Can you work these out from the model? Positions are in its coordinate system, mm. A direction names the side the tool comes from. Round coordinates to 2 decimals unless told otherwise and drop trailing zeros. Order: outer loops, then holes, each group sorted by start corner. A loop starts at its lowest first (then second) coordinate and runs counter-clockwise, first axis right, second up.
Q1. Will this pin go through, and if not, where does the flat tip stop? P1, Ø7.5, axis at y = 4, z = -81, coming from the -X side.
Q2. For faces 1 (the face through (-200, 10, 1)), 2 (the face through (-144, 10, 60)), which set-ups out of +Z, -Z, +X, -X, +Y, -Y let a thin tool reach every point of the face, with its end or its side?
Q3. If we section it at A-A (z = 0): Please give me the cut outline in (x, y), plus the area to 3 significant figures.
Q4. We'd pull the mould along Z, two halves only. Please class faces 3 (the face through (-1, 7, 100)), 4 (the face through (-144, 10, -60)), 5 (the face through (-100, 7, -80)), 6 (the face through (1.32, 7.4, -29.97)): pulls with the +Z half, pulls with the -Z half, needs draft (parallel to the pull), parting line crosses it, or undercut.
Q5. If I drill on line 1 (X direction, y = 7, z = 0); line 2 (X direction, y = 4.5, z = 84); line 3 (X direction, y = 3, z = 0), over which ranges is the centre line in solid material (lowest first)?
Q6. If we section it at B-B (z = -75.5): Please give me the cut outline in (x, y).
Q7. If we section it at C-C (x = -171.5): Please give me the cut outline in (y, z), plus the area to 3 significant figures.
from build123d import *

# Parameters (mm, degrees)
SKETCH2_W           = 200
SKETCH2_H           = 200
SKETCH2_R           = 30
BOSS_EXTRUDE2_DEPTH = 20
BOSS_EXTRUDE3_DEPTH = 100
FILLET1_R           = 5


with BuildPart() as part:
    # Sketch2 → Boss-Extrude2 (new body)
    with BuildSketch(Plane(origin=(0, 0, 0), x_dir=(1, 0, 0), z_dir=(0, 1, 0))):
        Rectangle(SKETCH2_W, SKETCH2_H)
        with Locations(Location((0, 0, 0), (0, 0, 270))):
            Circle(SKETCH2_R, mode=Mode.SUBTRACT)
    extrude(amount=BOSS_EXTRUDE2_DEPTH)

    # Sketch4 → Boss-Extrude3 (add)
    with BuildSketch(Plane.ZY.offset(100)):
        with BuildLine():
            Line((-50, 20), (50, 20))
            ThreePointArc((50, 20), (60, 10), (50, 0))
            Line((50, 0), (-50, 0))
            ThreePointArc((-50, 0), (-60, 10), (-50, 20))
        make_face()
    extrude(amount=BOSS_EXTRUDE3_DEPTH)

    # Fillet1
    fillet1_edges = [part.edges().sort_by_distance(p)[0] for p in [
        (0, 20, -30),
        (-100, 20, -75),
        (0, 20, 100),
        (-100, 20, 75),
        (-200, 10, -60),
        (-200, 0, 0),
        (-200, 10, 60),
        (-200, 20, 0),
        (100, 20, 0),
        (0, 20, -100),
    ]]
    fillet(fillet1_edges, radius=FILLET1_R)


solid = part.part
Solution:
1. P1: stops at x = -100
2. face 1: +Z, -Z, -X, +Y, -Y
2. face 2: +Z, -X
3. outline: (-200, 5) arc R5 ccw to (-195, 0) - (-30, 0) - (-30, 15) arc R5 ccw to (-35, 20) - (-195, 20) arc R5 ccw to (-200, 15) - close; (30, 0) - (100, 0) - (100, 15) arc R5 ccw to (95, 20) - (35, 20) arc R5 ccw to (30, 15) - close
3. area: 4,770 mm2
4. face 3: pulls with the +Z half
4. face 4: pulls with the -Z half
4. face 5: needs draft
4. face 6: undercut
5. line 1: x = -200 to -30, 30 to 100
5. line 2: x = -100 to 100
5. line 3: x = -199.58 to -30, 30 to 100
6. outline: (-100, 0) - (100, 0) - (100, 15) arc R5 ccw to (95, 20) - (-95, 20) arc R5 ccw to (-100, 15) - close
7. outline: (0, -50) arc R10 ccw to (20, -50) - (20, 50) arc R10 ccw to (0, 50) - close
7. area: 2,310 mm2
